from build123d import *

# Parameters (mm, degrees)
EXTRUDE_1_DEPTH     = 40
SKETCH_8_R          = 2
CUT_EXTRUDE_5_DEPTH = 50


with BuildPart() as part:
    # Эскиз1 → Бобышка-Вытянуть1 (new body)
    with BuildSketch(Plane.XY):
        with BuildLine():
            Line((0, 0), (100, 0))
            Line((100, 0), (100, 34))
            Line((100, 34), (100, 50))
            Line((100, 50), (0, 50))
            Line((0, 50), (0, 26))
            Line((0, 26), (12.566965626, 26))
            ThreePointArc((12.566965626, 26), (27.5, 25), (12.566965626, 24))
            Line((12.566965626, 24), (0, 24))
            Line((0, 24), (0, 0))
        make_face()
        with BuildLine():
            Line((52.566965626, 26), (40, 26))
            Line((40, 26), (40, 24))
            Line((40, 24), (52.566965626, 24))
            ThreePointArc((52.566965626, 24), (60, 17.5), (67.433034374, 24))
            Line((67.433034374, 24), (80, 24))
            Line((80, 24), (80, 26))
            Line((80, 26), (67.433034374, 26))
            ThreePointArc((67.433034374, 26), (60, 32.5), (52.566965626, 26))
        make_face(mode=Mode.SUBTRACT)
    extrude(amount=EXTRUDE_1_DEPTH)

    # Эскиз8 → Вырез-Вытянуть5 (cut)
    with BuildSketch(Plane.XZ):
        with Locations(Location((8, 30, 0), (0, 0, 270))):
            Circle(SKETCH_8_R)
        with Locations(Location((8, 10, 0), (0, 0, 270))):
            Circle(SKETCH_8_R)
        with Locations(Location((48, 30, 0), (0, 0, 270))):
            Circle(SKETCH_8_R)
        with Locations(Location((48, 10, 0), (0, 0, 270))):
            Circle(SKETCH_8_R)
    extrude(amount=-CUT_EXTRUDE_5_DEPTH, mode=Mode.SUBTRACT)


solid = part.part
Geometry: final body of the model. Coordinates: model frame, mm. A direction names the side the tool comes from. Coordinates: 2 decimals unless noted, no trailing zeros. Loops run counter-clockwise (first coordinate to the right, second up) from the corner with the lowest first, then second, coordinate; pieces in that order, holes last. Notation, with made-up numbers: (-14, 48.5) - (-4, 48.5) arc R14 cw to (-4, 75.5) - close; hole circle Ø4 at (-32, 89). An arc over 180 degrees is marked (long way). Put each result on its own line as item: value. Start each with the question number.
Q1. Line query: line 1 (X direction, y = 10, z = 10); line 2 (Y direction, x = 68, z = 18.5); line 3 (X direction, y = 29.5, z = 25). Output: solid intervals per line, ascending.
Q2. Pull-direction query (Y, two-part tool) for faces 1 (the flat face through (51, 50, 20)), 2 (the cylindrical face through (46.226, 11.832, 29.077)), 3 (the flat face through (46, 24, 20)); classes: released by +Y, released by -Y, zero draft, split by the parting line, or undercut.
Q3. Cut plane A-A, the plane z = 30. Give the number of separate pieces and of enclosed holes in the cut face, and give its area (3 significant figures).
Q4. Pin query (flat end, axial travel): pin 1 Ø3 at (x, z) = (48, 30) entering from -Y; pin 2 Ø12 at (y, z) = (26, 12.5) entering from -X. Return the tip coordinate at first contact, or that it passes through.
Q5. Cut plane D-D, the plane z = 3. Return loops of the section in (x, y).
Q6. Cut plane B-B, the plane y = 30.5. Return loops of the section in (x, z).
Q7. Set-up query: faces 4 (the cylindrical face through (46, 12, 10)), 5 (the flat face through (40, 25, 20)). Return all of +Z, -Z, +X, -X, +Y, -Y with unobstructed straight access to the full face (end or side cutting, diameter ignored); none if empty.
Q8. Cut plane C-C, the plane x = 20. Return loops of the section in (y, z), and give its area (3 significant figures).
Filled sheet:
1. line 1: 0 to 6, 10 to 46, 50 to 100
1. line 2: 0 to 24, 26 to 50
1. line 3: 0 to 14, 26 to 54, 66 to 100
2. face 1: released by +Y
2. face 2: zero draft
2. face 3: undercut
3. separate pieces: 4
3. enclosed holes: 0
3. area: 4,190 mm²
4. pin 1: through
4. pin 2: x = 0
5. outline: (0, 0) - (100, 0) - (100, 50) - (0, 50) - (0, 26) - (12.57, 26) arc R7.5 cw (long way) to (12.57, 24) - (0, 24) - close; hole (40, 24) - (52.57, 24) arc R7.5 ccw to (67.43, 24) - (80, 24) - (80, 26) - (67.43, 26) arc R7.5 ccw to (52.57, 26) - (40, 26) - close
6. outline: (0, 0) - (14.9, 0) - (14.9, 40) - (0, 40) - close; (25.1, 0) - (54.9, 0) - (54.9, 40) - (25.1, 40) - close; (65.1, 0) - (100, 0) - (100, 40) - (65.1, 40) - close; hole circle Ø4 at (8, 10); hole circle Ø4 at (8, 30); hole circle Ø4 at (48, 10); hole circle Ø4 at (48, 30)
7. face 4: +Y, -Y
7. face 5: +Z, -Z
8. outline: (0, 0) - (17.5, 0) - (17.5, 40) - (0, 40) - close; (32.5, 0) - (50, 0) - (50, 40) - (32.5, 40) - close
8. area: 1,400 mm²
